from build123d import *

# Parameters (mm, degrees)
BOSS_EXTRU_1_DEPTH      = 10
CONG_3_R                = 5
CONG_4_R                = 5
CONG_5_R                = 1
CONG_6_R                = 1
ENL_V_MAT_EXTRU_1_DEPTH = 30


with BuildPart() as part:
    # Esquisse1 → Boss.-Extru.1 (new body)
    with BuildSketch(Plane(origin=(0, 0, 0), x_dir=(1, 0, 0), z_dir=(0, 1, 0))):
        Polygon((50, 30), (50, 5), (-50, 5), (-50, -5), (50, -5), (50, -30), (60, -30), (60, 30), align=None)
    extrude(amount=BOSS_EXTRU_1_DEPTH)

    # Congé3
    cong_3_edges = [part.edges().sort_by_distance(p)[0] for p in [
        (60, 5, 30),
        (50, 5, 30),
    ]]
    fillet(cong_3_edges, radius=CONG_3_R - 0.0001)  # a hair under: the kernel refuses the full size

    # Congé4
    cong_4_edges = [part.edges().sort_by_distance(p)[0] for p in [
        (-50, 5, 5),
        (-50, 5, -5),
    ]]
    fillet(cong_4_edges, radius=CONG_4_R - 0.0001)  # a hair under: the kernel refuses the full size

    # Congé5
    cong_5_edges = [part.edges().sort_by_distance(p)[0] for p in [
        (50, 5, -30),
    ]]
    fillet(cong_5_edges, radius=CONG_5_R)

    # Congé6
    cong_6_edges = [part.edges().sort_by_distance(p)[0] for p in [
        (60, 5, -30),
    ]]
    fillet(cong_6_edges, radius=CONG_6_R)

    # Esquisse3D1 → Enlèv. mat.-Extru.1 (cut)
    with BuildSketch(Plane(origin=(-50, 4.5, -1.5), x_dir=(0, 0.3162277660168382, 0.9486832980505138), z_dir=(-1, 0, 0))):
        Polygon((0, 0), (2.846049894, -0.948683298), (3.16227766, 0), (0.316227766, 0.948683298), align=None)
    extrude(amount=-ENL_V_MAT_EXTRU_1_DEPTH, mode=Mode.SUBTRACT)


solid = part.part
Verification items for the finished model (mm, model axes). A direction names the side the tool comes from. Coordinates: 2 decimals unless noted, no trailing zeros. Write each loop counter-clockwise with the first axis right and the second up, starting at its lowest first coordinate (ties: lowest second). Pieces come first, ordered by that corner, then holes. Notation, with made-up numbers: M 12.25,-37.75 L 47.25,-37.75 A28 ccw 47.25,-2.75 Z; hole C 59.5,24 d9. An arc over 180 degrees is marked long. Use CSV: the item, a comma, the result in double quotes.
Q1. Go/stop test with flat-tipped pins: P1, Ø2.5, axis at x = -34, z = 0.5, coming from the -Y side; P2, Ø6, axis at x = -31, y = 5, coming from the +Z side; P3, Ø0.5, axis at x = -41, y = 5, coming from the -Z side; P4, Ø0.8, axis at y = 5, z = -0.5, coming from the -X side. Record where each tip stops, or that it passes through.
Computed values:
P1,"y = 0"
P2,"z = 5"
P3,"z = -5"
P4,"x = -20"
Q2. Section check D-D, the plane z = -15. Enter the section's corners in (x, y).
Computed values:
outline,"M 50,0 L 60,0 L 60,10 L 50,10 Z"
Q3. Mould release check, pull along Y, two halves, no side actions. Record for faces 1 (the flat face through (-35, 5.5, 0)), 2 (the flat face through (17, 0, 2)), 3 (the cylindrical face through (58, 5, 29)): pulls with the +Y half, pulls with the -Y half, needs draft (parallel to the pull), parting line crosses it, or undercut.
Computed values:
face 1,"undercut"
face 2,"pulls with the -Y half"
face 3,"needs draft"
Q4. Section check A-A, the plane x = -43. Enter the section's corners in (y, z).
Computed values:
outline,"M 0,-5 L 10,-5 L 10,5 L 0,5 Z; hole M 4.5,-1.5 L 5.5,-1.5 L 5.5,1.5 L 4.5,1.5 Z"
Q5. Set-up check for faces 4 (the flat face through (2, 5, 5)), 5 (the flat face through (17, 10, 2)), 6 (the flat face through (3, 5, -5)), 7 (the flat face through (-35, 4.5, 0)): record each of +Z, -Z, +X, -X, +Y, -Y from which the full face is reachable in a straight line by a thin tool's end or side.
Computed values:
face 4,"+Z, -X, +Y, -Y"
face 5,"+Z, -Z, +X, -X, +Y"
face 6,"-Z, -X, +Y, -Y"
face 7,"-X"
Q6. Section check C-C, the plane x = -7.5. Enter the section's corners in (y, z).
Computed values:
outline,"M 0,-5 L 10,-5 L 10,5 L 0,5 Z"
Q7. Thickness scan on line 1 along X through (y, z) = (8, 25.5); line 2 along Z through (x, y) = (-18.5, 2.5); line 3 along X through (y, z) = (7, -3). Record the ranges inside material, lowest first. Write a range as [from, to].
Computed values:
line 1,"[50.03, 59.97]"
line 2,"[-5, 5]"
line 3,"[-49, 60]"
